```python
from build123d import *

# Parameters (mm, degrees)
SKETCH1_W            = 165.1
SKETCH1_H            = 139.7
BOSS_EXTRUDE1_DEPTH  = 9.525
SKETCH2_W            = 50.8
SKETCH2_H            = 50.8
BOSS_EXTRUDE2_DEPTH  = 63.5
FILLET1_R            = 25.4
FILLET1_OF_MIRROR1_R = 25.4
SKETCH5_R            = 19.05
BASE_HOLE_DEPTH      = 126.402452129


with BuildPart() as part:
    # Sketch1 → Boss-Extrude1 (new body)
    with BuildSketch(Plane(origin=(0, 0, 0), x_dir=(1, 0, 0), z_dir=(0, 1, 0))):
        Rectangle(SKETCH1_W, SKETCH1_H)
    extrude(amount=BOSS_EXTRUDE1_DEPTH)

    # Sketch2 → Boss-Extrude2 (add)
    with BuildSketch(Plane(origin=(0, 9.525, 0), x_dir=(1, 0, 0), z_dir=(0, 1, 0))):
        with Locations((-57.15, 44.45)):
            Rectangle(SKETCH2_W, SKETCH2_H)
    boss_extrude2 = extrude(amount=BOSS_EXTRUDE2_DEPTH)

    # Sketch3 → 1/2-20 Tapped Hole1 (revolve, cut)
    with BuildSketch(Plane(origin=(-57.15, 73.025, -44.45), x_dir=(0, 0, 1), z_dir=(1, 0, 0))):
        Polygon((0, 0), (0, 35.20757432), (5.75437, 31.75), (5.75437, 0), align=None)
    f_1_2_20_tapped_hole1 = revolve(axis=Axis((-57.15, 79.375, -44.45), (0, -1, 0)), mode=Mode.SUBTRACT)

    # Fillet1
    fillet1_edges = [part.edges().sort_by_distance(p)[0] for p in [
        (-31.75, 41.275, -19.05),
    ]]
    fillet(fillet1_edges, radius=FILLET1_R)

    # Mirror1: Boss-Extrude2, 1/2-20 Tapped Hole1 across plane
    add(boss_extrude2.mirror(Plane(origin=(0, 0, 0), x_dir=(0, 0, 1), z_dir=(1, 0, 0))))
    add(f_1_2_20_tapped_hole1.mirror(Plane(origin=(0, 0, 0), x_dir=(0, 0, 1), z_dir=(1, 0, 0))), mode=Mode.SUBTRACT)

    # Fillet1 of Mirror1
    fillet1_of_mirror1_edges = [part.edges().sort_by_distance(p)[0] for p in [
        (31.75, 41.275, -19.05),
    ]]
    fillet(fillet1_of_mirror1_edges, radius=FILLET1_OF_MIRROR1_R)

    # Sketch5 → base hole (cut, through all)
    with BuildSketch(Plane(origin=(0, 9.525, 0), x_dir=(1, 0, 0), z_dir=(0, 1, 0))):
        with Locations(Location((0, 0, 0), (0, 0, 270))):
            Circle(SKETCH5_R)
    extrude(amount=-BASE_HOLE_DEPTH, mode=Mode.SUBTRACT)


solid = part.part
```
Geometry check sheet. Reference: the model listing, model coordinates, mm. A direction names the side the tool comes from. Coordinates: 2 decimals unless noted, no trailing zeros. Loops run counter-clockwise (first coordinate to the right, second up) from the corner with the lowest first, then second, coordinate; pieces in that order, holes last. Notation, with made-up numbers: (82.5, 86) -> (138.5, 86) arc R16 cw to (138.5, 94) -> close; hole circle Ø10 at (40, 75). An arc over 180 degrees is marked (long way). Put each result on its own line as item: value.
1) Cross-section at A-A on y = 67.5. Record the boundary of the cut face in (x, z).
Result set:
outline: (-82.55, -69.85) -> (-31.75, -69.85) -> (-31.75, -44.45) arc R25.4 ccw to (-57.15, -19.05) -> (-82.55, -19.05) -> close; (31.75, -69.85) -> (82.55, -69.85) -> (82.55, -19.05) -> (57.15, -19.05) arc R25.4 ccw to (31.75, -44.45) -> close; hole circle Ø11.51 at (-57.15, -44.45); hole circle Ø11.51 at (57.15, -44.45)
2) Cross-section at D-D on x = -7. Record the boundary of the cut face in (y, z) (3 decimals).
Result set:
outline: (0, -69.85) -> (9.525, -69.85) -> (9.525, -17.717) -> (0, -17.717) -> close; (0, 17.717) -> (9.525, 17.717) -> (9.525, 69.85) -> (0, 69.85) -> close
3) Gauge pin test, flat ends, axial feed: pin 1 Ø10.5 at (x, z) = (-57.15, -44.45) entering from -Y; pin 2 Ø20.5 at (x, y) = (-72, 56) entering from +Z; pin 3 Ø10 at (x, y) = (40.5, 49) entering from +Z; pin 4 Ø7.5 at (x, y) = (75.5, 43) entering from +Z. Record the tip position at first contact, or that the pin passes through.
Result set:
pin 1: stops at y = 0
pin 2: stops at z = -19.05
pin 3: stops at z = -21.88
pin 4: stops at z = -19.05
4) Cross-section at C-C on y = 24. Record the boundary of the cut face in (x, z).
Result set:
outline: (-82.55, -69.85) -> (-31.75, -69.85) -> (-31.75, -44.45) arc R25.4 ccw to (-57.15, -19.05) -> (-82.55, -19.05) -> close; (31.75, -69.85) -> (82.55, -69.85) -> (82.55, -19.05) -> (57.15, -19.05) arc R25.4 ccw to (31.75, -44.45) -> close
5) Thickness scan on line 1 (X direction, y = 61, z = -44); line 2 (Z direction, x = -57, y = 54); line 3 (X direction, y = 54, z = -61.5). Record the ranges inside material, lowest first.
Result set:
line 1: x = -82.55 to -62.89, -51.41 to -31.75, 31.75 to 51.41, 62.89 to 82.55
line 2: z = -69.85 to -50.2, -38.7 to -19.05
line 3: x = -82.55 to -31.75, 31.75 to 82.55
6) Tool access check on faces 1 (the cylindrical face through (-52.045, 57.372, -41.795)), 2 (the flat face through (-70, 41, -19.05)), 3 (the flat face through (-1, 9.525, 30)), 4 (the flat face through (31.75, 41, -57)). Record the directions out of +Z, -Z, +X, -X, +Y, -Y that give a thin tool (end or side, any length) a straight path to the whole face; none if there is none.
Result set:
face 1: +Y
face 2: +Z, +X, -X, +Y
face 3: +Z, +Y
face 4: +Z, -Z, +Y
7) Release check for a two-part mould opening along Z. For faces 5 (the cylindrical face through (39.39, 41.72, -26.29)), 6 (the cylindrical face through (52.045, 57.372, -41.795)), 7 (the flat face through (-31.75, 41, -57)), 8 (the conical face through (-56.26, 38.42, -43.99)) record: released by +Z, released by -Z, zero draft, split by the parting line, or undercut.
Result set:
face 5: released by +Z
face 6: undercut
face 7: zero draft
face 8: undercut
8) Cross-section at B-B on z = 0. Record the boundary of the cut face in (x, y) (3 decimals), plus the area to 3 significant figures.
Result set:
outline: (-82.55, 0) -> (-19.05, 0) -> (-19.05, 9.525) -> (-82.55, 9.525) -> close; (19.05, 0) -> (82.55, 0) -> (82.55, 9.525) -> (19.05, 9.525) -> close
area: 1,210 mm^2
